For this review, take the finished solid that the model builds, in its own axes (mm). Round coordinates to 2 decimals unless told otherwise and drop trailing zeros. Order: outer loops, then holes, each group sorted by start corner. A loop starts at its lowest first (then second) coordinate and runs counter-clockwise, first axis right, second up. Notation, with made-up numbers: (89, 9) - (126, 9) arc R25 cw to (126, 39) - close; hole circle Ø6 at (26.25, 37). An arc over 180 degrees is marked (long way). Write each question's results on one line, items separated by ' | '. Start each with the question number.
(1) Insertion check: pin 1 Ø16 at (x, z) = (-0.02, -2.43) entering from +Y. The pin has a flat end and moves straight along its axis. Give the tip position at first contact, or say it passes through.
(2) Take a section at C-C, the plane x = -8.5. Give the boundary of the cut face in (y, z), plus the area to 3 significant figures.
(3) Take a section at D-D, the plane z = -11. Give the boundary of the cut face in (x, y).
(4) Take a section at B-B, the plane z = 14. Give the boundary of the cut face in (x, y), plus the area to 3 significant figures.
(5) Take a section at A-A, the plane x = 3.5. Give the boundary of the cut face in (y, z).
(6) For L1, parallel to X at y = 0.8, z = 15.5; L2, parallel to Z at x = -7, y = 1.25; L3, parallel to Z at x = 8.25, y = 0.65, list the stretches that pass through material, from the lowest coordinate up. Write a range as from..to.
Autodesk Inventor part; units mm, degrees
ref_plane "YZ Plane" through (0, 0, 0) normal (1, 0, 0) x (0, 1, 0)
ref_plane "XZ Plane" through (0, 0, 0) normal (0, 1, 0) x (-1, 0, 0)
ref_plane "XY Plane" through (0, 0, 0) normal (0, 0, 1) x (1, 0, 0)
sketch "Sketch1" plane through (0, 0, 0) normal (0, 1, 0) x (-1, 0, 0)
  arc A0 (-14.8294, -2.4305) -> (14.8706, -2.4305) centre (0.0206, -2.4305) ccw
  line L0 (14.8706, 17.5695) -> (-14.8294, 17.5695)
  line L1 (14.8706, -2.4305) -> (14.8706, 17.5695)
  line L2 (14.8706, 17.5695) -> (-14.8294, 17.5695)
  line L3 (-14.8294, 17.5695) -> (-14.8294, -2.4305)
  circle A1 centre (0.0206, -2.4305) radius 10
  line L4 (0.0206, 17.5695) -> (0.0206, 7.5695)
  line L5 (0.0206, 17.5695) -> (0.0206, 15.0695)
  line L6 (-14.8294, 15.0695) -> (0.0206, 15.0695)
  line L7 (1.5206, 17.5695) -> (1.5206, 12.5695)
  line L8 (0.0206, 15.0695) -> (14.8706, 15.0695)
  circle A2 centre (-7.4044, 15.0695) radius 1.5
  circle A3 centre (7.4456, 15.0695) radius 1.5
  point P0 (0, 0)
  dimension "d0" = 20
  dimension "d1" = 3
  dimension "d2" = 3
extrude "Extrusion1" add sketch "Sketch1" along normal blind 2 contours L3 L6 A2 L8 A3 L1 A0 | L3 L0 L4 L6 A2 | L8 A3 L7 L0 L1 | L0 L7 L8 L4
thread "Thread1"
thread "Thread2"
properties part number "Holder Cover"
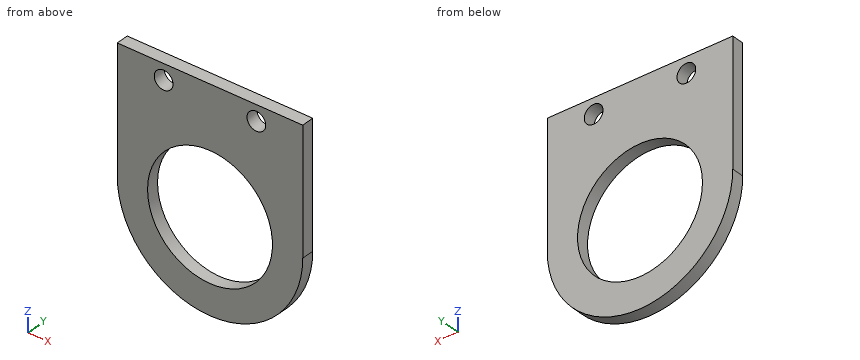
Results below:
1) pin 1: passes through
2) outline: (0, -14.62) - (2, -14.62) - (2, -7.73) - (0, -7.73) - close; (0, 2.87) - (2, 2.87) - (2, 14) - (0, 14) - close; (0, 16.14) - (2, 16.14) - (2, 17.57) - (0, 17.57) - close | area: 38.9 mm^2
3) outline: (-12.15, 0) - (-5.17, 0) - (-5.17, 2) - (-12.15, 2) - close; (5.13, 0) - (12.11, 0) - (12.11, 2) - (5.13, 2) - close
4) outline: (-14.87, 0) - (-8.5, 0) - (-8.5, 2) - (-14.87, 2) - close; (-6.39, 0) - (6.35, 0) - (6.35, 2) - (-6.39, 2) - close; (8.46, 0) - (14.83, 0) - (14.83, 2) - (8.46, 2) - close | area: 51.0 mm^2
5) outline: (0, -16.86) - (2, -16.86) - (2, -11.79) - (0, -11.79) - close; (0, 6.93) - (2, 6.93) - (2, 17.57) - (0, 17.57) - close
6) L1: x = -14.87..-8.88, -6.01..5.97, 8.84..14.83 | L2: z = -15.54..-9.59, 4.73..13.64, 16.5..17.57 | L3: z = -14.76..-8.05, 3.19..13.83, 16.31..17.57
